Here's how the part is built. I have some questions about the finished solid (model axes, mm). Round coordinates to 2 decimals unless told otherwise and drop trailing zeros. Write each loop counter-clockwise with the first axis right and the second up, starting at its lowest first coordinate (ties: lowest second). Pieces come first, ordered by that corner, then holes. Notation, with made-up numbers: (30.25, 70.25) - (83.25, 70.25) arc R19 ccw to (83.25, 83.25) - close; hole circle Ø9 at (-37.75, 8). An arc over 180 degrees is marked (long way). Write item = value, one per line. Start each with the question number.
Item 1: If I drill on line 1 along Y through (x, z) = (168, 8.5); line 2 along Y through (x, z) = (240.5, 4.75); line 3 along Z through (x, y) = (-268, -16.5), over which ranges is the centre line in solid material (lowest first)? Write a range as [from, to].
Item 2: If we section it at B-B (z = 3.75): Please give me the cut outline in (x, y).
Item 3: If we section it at A-A (x = 173): Please give me the cut outline in (y, z).
```python
from build123d import *

# Parameters (mm, degrees)
F0_W     = 50
F0_H     = 10
F1_DEPTH = 301.5
F2_SIZE  = 9


with BuildPart() as f1:
    # F0 (on Right) → F1 (new body, symmetric)
    with BuildSketch(Plane.YZ):
        with Locations((0, 5)):
            Rectangle(F0_W, F0_H)
    extrude(amount=F1_DEPTH, both=True)

    # F2
    f2_edges = [f1.edges().sort_by_distance(p)[0] for p in [
        (0, -25, 10),
    ]]
    chamfer(f2_edges, length=F2_SIZE)


solid = f1.part
```
Reply:
q1.line_1 = [-17.5, 25]
q1.line_2 = [-21.25, 25]
q1.line_3 = [0, 9.5]
q2.outline = (-301.5, -22.25) - (301.5, -22.25) - (301.5, 25) - (-301.5, 25) - close
q3.outline = (-25, 0) - (25, 0) - (25, 10) - (-16, 10) - (-25, 1) - close
